Can you work these out from the model? Positions are in its coordinate system, mm. A direction names the side the tool comes from. Round coordinates to 2 decimals unless told otherwise and drop trailing zeros. Write each loop counter-clockwise with the first axis right and the second up, starting at its lowest first coordinate (ties: lowest second). Pieces come first, ordered by that corner, then holes. Notation, with made-up numbers: M -28,-12.5 L 12,-12.5 A29 ccw 12,26.5 Z; hole C 85.5,41 d3. An arc over 180 degrees is marked long. Answer as a JSON object with one key per item and string values. Group by question number.
1) On a 3-axis mill with a long thin cutter (end or side, diameter ignored), from which of +Z, -Z, +X, -X, +Y, -Y can I reach the whole of each face in a straight line? I mean faces 4 (the flat face through (-15, -62, 2)), 5 (the flat face through (-37, 60, 2)), 6 (the flat face through (-5, 62, 2)), 7 (the flat face through (37, -60, 2)), 8 (the flat face through (60, 37, 2)). Say none if no direction works.
2) I'm going to push flat-ended pins straight in: pin 1 Ø1.5 at (y, z) = (61.5, 2.5) entering from -X; pin 2 Ø2.5 at (y, z) = (-63, 3) entering from +X; pin 3 Ø2.5 at (x, z) = (39, 3.5) entering from -Y; pin 4 Ø3 at (x, y) = (15.5, -15.5) entering from -Z. Where does each tip first touch, or does it pass through?
3) Please list where these lines run through material, in increasing order: L1, parallel to Y at x = -15.5, z = 3.8; L2, parallel to Y at x = 0, z = 1.55; L3, parallel to Y at x = -54.5, z = 3.8. Write a range as [from, to].
4) Suppose I cut it at A-A, the plane y = 0. Write out the boundary of the cut face in (x, z), and give its area (4 significant figures).
5) If we mould it in two halves opening along X, with no side actions, what happens to faces 1 (the flat face through (-60, 0, 2)), 2 (the flat face through (65, 10, 2)), 3 (the flat face through (0, -60, 2))? For each: +X half, -X half, draft (parallel to the pull), parting line (faces both ways), or undercut.
6) Suppose I cut it at D-D, the plane y = 37. Write out the boundary of the cut face in (x, z), and give its area (3 significant figures).
7) Suppose I cut it at C-C, the plane z = 0.85. State how many separate pieces and enclosed holes the cut face has, and give its area (3 significant figures).
from build123d import *

# Parameters (mm, degrees)
SKETCH1_R           = 11.25
SKETCH1_R_2         = 1.8
BOSS_EXTRUDE1_DEPTH = 5


with BuildPart() as part:
    # Sketch1 → Boss-Extrude1 (new body)
    with BuildSketch(Plane.XY):
        Polygon((5, 60), (-5, 60), (-5, 65), (-15, 65), (-15, 60), (-60, 60), (-60, 15), (-65, 15), (-65, 5), (-60, 5), (-60, -5), (-65, -5), (-65, -15), (-60, -15), (-60, -60), (-15, -60), (-15, -65), (-5, -65), (-5, -60), (5, -60), (5, -65), (15, -65), (15, -60), (60, -60), (60, -15), (65, -15), (65, -5), (60, -5), (60, 5), (65, 5), (65, 15), (60, 15), (60, 60), (15, 60), (15, 65), (5, 65), align=None)
        Circle(SKETCH1_R, mode=Mode.SUBTRACT)
        with Locations((-15.5, 15.5)):
            Circle(SKETCH1_R_2, mode=Mode.SUBTRACT)
        with Locations((15.5, 15.5)):
            Circle(SKETCH1_R_2, mode=Mode.SUBTRACT)
        with Locations((15.5, -15.5)):
            Circle(SKETCH1_R_2, mode=Mode.SUBTRACT)
        with Locations((-15.5, -15.5)):
            Circle(SKETCH1_R_2, mode=Mode.SUBTRACT)
    extrude(amount=BOSS_EXTRUDE1_DEPTH)


solid = part.part
Results:
{
 "1": {"face 4": "+Z, -Z, -X, -Y", "face 5": "+Z, -Z, -X, +Y", "face 6": "+Z, -Z, +Y", "face 7": "+Z, -Z, +X, -Y", "face 8": "+Z, -Z, +X, +Y"},
 "2": {"pin 1": "x = -15", "pin 2": "x = 15", "pin 3": "y = -60", "pin 4": "through"},
 "3": {"L1": "[-60, -17.3], [-13.7, 13.7], [17.3, 60]", "L2": "[-60, -11.25], [11.25, 60]", "L3": "[-60, 60]"},
 "4": {"outline": "M -60,0 L -11.25,0 L -11.25,5 L -60,5 Z; M 11.25,0 L 60,0 L 60,5 L 11.25,5 Z", "area": "487.5 mm^2"},
 "5": {"face 1": "-X half", "face 2": "+X half", "face 3": "undercut"},
 "6": {"outline": "M -60,0 L 60,0 L 60,5 L -60,5 Z", "area": "600 mm^2"},
 "7": {"separate pieces": "1", "enclosed holes": "5", "area": "14,400 mm^2"}
}
